Source: CAD feature listing. Evaluate the final solid. Frame: model axes, mm. Give positions to 0.01 mm unless a question says otherwise; leave off trailing zeros. Loops run counter-clockwise (first coordinate to the right, second up) from the corner with the lowest first, then second, coordinate; pieces in that order, holes last. Notation, with made-up numbers: (-1, 81.25) -> (21, 81.25) arc R20 cw to (21, 103.25) -> close; hole circle Ø4 at (1.25, 68). An arc over 180 degrees is marked (long way). Put each result on its own line as item: value.
```python
from build123d import *

# Parameters (mm, degrees)
SKETCH1_W           = 710
SKETCH1_H           = 275
SKETCH1_R           = 22.5
BOSS_EXTRUDE1_DEPTH = 3


with BuildPart() as part:
    # Sketch1 → Boss-Extrude1 (new body)
    with BuildSketch(Plane(origin=(0, 0, 0), x_dir=(1, 0, 0), z_dir=(0, 1, 0))):
        with Locations((355, 0)):
            Rectangle(SKETCH1_W, SKETCH1_H)
        with Locations((23, 100.9)):
            Circle(SKETCH1_R, mode=Mode.SUBTRACT)
        with Locations((23, 49.9)):
            Circle(SKETCH1_R, mode=Mode.SUBTRACT)
        with Locations((23, -49.9)):
            Circle(SKETCH1_R, mode=Mode.SUBTRACT)
        with Locations((23, -100.9)):
            Circle(SKETCH1_R, mode=Mode.SUBTRACT)
        with Locations((78.35, 100.9)):
            Circle(SKETCH1_R, mode=Mode.SUBTRACT)
        with Locations((78.35, 49.9)):
            Circle(SKETCH1_R, mode=Mode.SUBTRACT)
        with Locations((78.35, -49.9)):
            Circle(SKETCH1_R, mode=Mode.SUBTRACT)
        with Locations((78.35, -100.9)):
            Circle(SKETCH1_R, mode=Mode.SUBTRACT)
        with Locations((133.7, 100.9)):
            Circle(SKETCH1_R, mode=Mode.SUBTRACT)
        with Locations((133.7, 49.9)):
            Circle(SKETCH1_R, mode=Mode.SUBTRACT)
        with Locations((133.7, -49.9)):
            Circle(SKETCH1_R, mode=Mode.SUBTRACT)
        with Locations((133.7, -100.9)):
            Circle(SKETCH1_R, mode=Mode.SUBTRACT)
        with Locations((189.05, 100.9)):
            Circle(SKETCH1_R, mode=Mode.SUBTRACT)
        with Locations((189.05, 49.9)):
            Circle(SKETCH1_R, mode=Mode.SUBTRACT)
        with Locations((189.05, -49.9)):
            Circle(SKETCH1_R, mode=Mode.SUBTRACT)
        with Locations((189.05, -100.9)):
            Circle(SKETCH1_R, mode=Mode.SUBTRACT)
        with Locations((244.4, 100.9)):
            Circle(SKETCH1_R, mode=Mode.SUBTRACT)
        with Locations((244.4, 49.9)):
            Circle(SKETCH1_R, mode=Mode.SUBTRACT)
        with Locations((244.4, -49.9)):
            Circle(SKETCH1_R, mode=Mode.SUBTRACT)
        with Locations((244.4, -100.9)):
            Circle(SKETCH1_R, mode=Mode.SUBTRACT)
        with Locations((299.75, 100.9)):
            Circle(SKETCH1_R, mode=Mode.SUBTRACT)
        with Locations((299.75, 49.9)):
            Circle(SKETCH1_R, mode=Mode.SUBTRACT)
        with Locations((299.75, -49.9)):
            Circle(SKETCH1_R, mode=Mode.SUBTRACT)
        with Locations((299.75, -100.9)):
            Circle(SKETCH1_R, mode=Mode.SUBTRACT)
        with Locations((355.1, 100.9)):
            Circle(SKETCH1_R, mode=Mode.SUBTRACT)
        with Locations((355.1, 49.9)):
            Circle(SKETCH1_R, mode=Mode.SUBTRACT)
        with Locations((355.1, -49.9)):
            Circle(SKETCH1_R, mode=Mode.SUBTRACT)
        with Locations((355.1, -100.9)):
            Circle(SKETCH1_R, mode=Mode.SUBTRACT)
        with Locations((410.45, 100.9)):
            Circle(SKETCH1_R, mode=Mode.SUBTRACT)
        with Locations((410.45, 49.9)):
            Circle(SKETCH1_R, mode=Mode.SUBTRACT)
        with Locations((410.45, -49.9)):
            Circle(SKETCH1_R, mode=Mode.SUBTRACT)
        with Locations((410.45, -100.9)):
            Circle(SKETCH1_R, mode=Mode.SUBTRACT)
        with Locations((465.8, 100.9)):
            Circle(SKETCH1_R, mode=Mode.SUBTRACT)
        with Locations((465.8, 49.9)):
            Circle(SKETCH1_R, mode=Mode.SUBTRACT)
        with Locations((465.8, -49.9)):
            Circle(SKETCH1_R, mode=Mode.SUBTRACT)
        with Locations((465.8, -100.9)):
            Circle(SKETCH1_R, mode=Mode.SUBTRACT)
        with Locations((521.15, 100.9)):
            Circle(SKETCH1_R, mode=Mode.SUBTRACT)
        with Locations((521.15, 49.9)):
            Circle(SKETCH1_R, mode=Mode.SUBTRACT)
        with Locations((521.15, -49.9)):
            Circle(SKETCH1_R, mode=Mode.SUBTRACT)
        with Locations((521.15, -100.9)):
            Circle(SKETCH1_R, mode=Mode.SUBTRACT)
        with Locations((576.5, 100.9)):
            Circle(SKETCH1_R, mode=Mode.SUBTRACT)
        with Locations((576.5, 49.9)):
            Circle(SKETCH1_R, mode=Mode.SUBTRACT)
        with Locations((576.5, -49.9)):
            Circle(SKETCH1_R, mode=Mode.SUBTRACT)
        with Locations((576.5, -100.9)):
            Circle(SKETCH1_R, mode=Mode.SUBTRACT)
        with Locations((631.85, 100.9)):
            Circle(SKETCH1_R, mode=Mode.SUBTRACT)
        with Locations((631.85, 49.9)):
            Circle(SKETCH1_R, mode=Mode.SUBTRACT)
        with Locations((631.85, -49.9)):
            Circle(SKETCH1_R, mode=Mode.SUBTRACT)
        with Locations((631.85, -100.9)):
            Circle(SKETCH1_R, mode=Mode.SUBTRACT)
        with Locations((687.2, 100.9)):
            Circle(SKETCH1_R, mode=Mode.SUBTRACT)
        with Locations((687.2, 49.9)):
            Circle(SKETCH1_R, mode=Mode.SUBTRACT)
        with Locations((687.2, -49.9)):
            Circle(SKETCH1_R, mode=Mode.SUBTRACT)
        with Locations((687.2, -100.9)):
            Circle(SKETCH1_R, mode=Mode.SUBTRACT)
    extrude(amount=BOSS_EXTRUDE1_DEPTH)


solid = part.part
```
(1) Section B-B on y = 1.45. Give the number of separate pieces and of enclosed holes in the cut face, then the cut area to 3 significant figures.
Calculated:
separate pieces: 1
enclosed holes: 52
area: 113,000 mm²
(2) Draft query along Z for faces 1 (the flat face through (350, 3, -2)), 2 (the cylindrical face through (201.1, 1.5, -119.9)). Return one class per face: released by +Z, released by -Z, zero draft, split by the parting line, or undercut.
Calculated:
face 1: zero draft
face 2: undercut
(3) Section A-A on x = 133.7. Return loops of the section in (y, z), then the cut area to 3 significant figures.
Calculated:
outline: (0, -137.5) -> (3, -137.5) -> (3, -123.4) -> (0, -123.4) -> close; (0, -78.4) -> (3, -78.4) -> (3, -72.4) -> (0, -72.4) -> close; (0, -27.4) -> (3, -27.4) -> (3, 27.4) -> (0, 27.4) -> close; (0, 72.4) -> (3, 72.4) -> (3, 78.4) -> (0, 78.4) -> close; (0, 123.4) -> (3, 123.4) -> (3, 137.5) -> (0, 137.5) -> close
area: 285 mm²
(4) Line query: probe 1 along Z at (x, y) = (576.5, 0.9); probe 2 along Z at (x, y) = (472, 2.45). Output: solid intervals per line, ascending. Write a range as from..to.
Calculated:
probe 1: z = -137.5..-123.4, -78.4..-72.4, -27.4..27.4, 72.4..78.4, 123.4..137.5
probe 2: z = -137.5..-122.53, -79.27..-71.53, -28.27..28.27, 71.53..79.27, 122.53..137.5
(5) Section D-D on x = 409.5. Return loops of the section in (y, z), then the cut area to 3 significant figures.
Calculated:
outline: (0, -137.5) -> (3, -137.5) -> (3, -123.38) -> (0, -123.38) -> close; (0, -78.42) -> (3, -78.42) -> (3, -72.38) -> (0, -72.38) -> close; (0, -27.42) -> (3, -27.42) -> (3, 27.42) -> (0, 27.42) -> close; (0, 72.38) -> (3, 72.38) -> (3, 78.42) -> (0, 78.42) -> close; (0, 123.38) -> (3, 123.38) -> (3, 137.5) -> (0, 137.5) -> close
area: 285 mm²
